Source: three-view drawing plus pictorial views. Frame: mm from the lowest corner of the part. Give positions to 0.01 mm unless a question says otherwise; leave off trailing zeros. Write each loop counter-clockwise with the first axis right and the second up, starting at its lowest first coordinate (ties: lowest second). Pieces come first, ordered by that corner, then holes. Notation, with made-up numbers: M 65,-2.75 L 112,-2.75 A28 ccw 112,23.25 Z; hole C -0.75,69 d11. An arc over 180 degrees is marked long. Return JSON: item names as keys, results as strings.
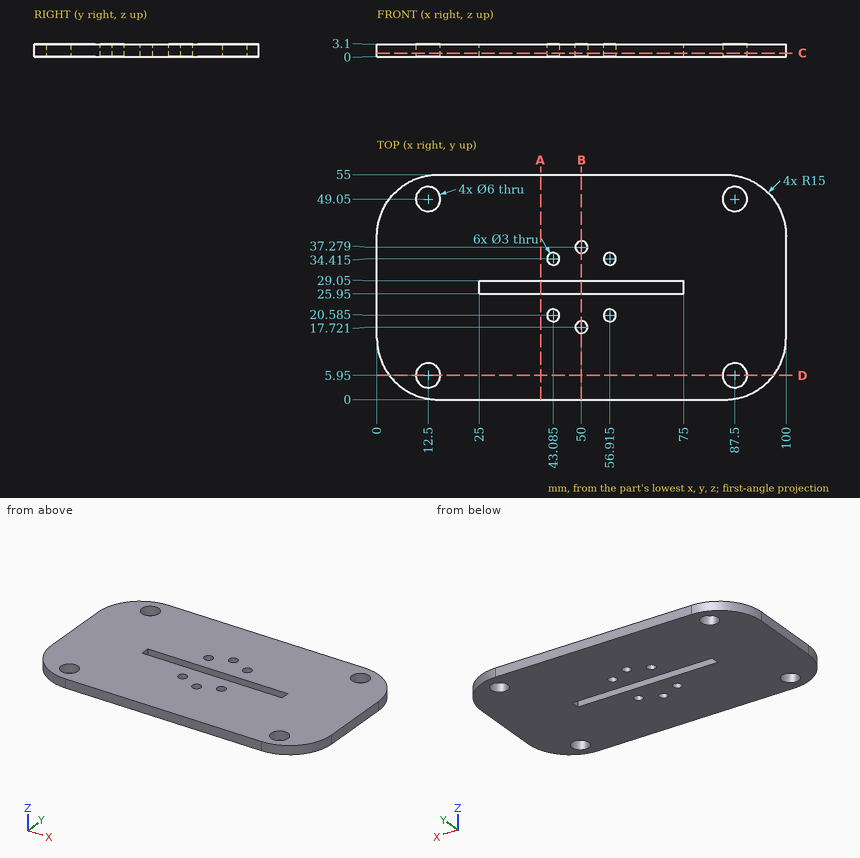
1) Contact query for a flat-ended pin moving along its axis: pin 1 Ø2.5 at (x, y) = (50, 17.721) entering from +Z. Output: stop coordinate, or through.
Numbers:
{"pin 1": "passes through"}
2) Cut plane B-B, the plane x = 50. Return the cut outline in (y, z).
Numbers:
{"outline": "M 0,0 L 16.22,0 L 16.22,3.1 L 0,3.1 Z; M 19.22,0 L 25.95,0 L 25.95,3.1 L 19.22,3.1 Z; M 29.05,0 L 35.78,0 L 35.78,3.1 L 29.05,3.1 Z; M 38.78,0 L 55,0 L 55,3.1 L 38.78,3.1 Z"}
3) Line query: line 1 (Y direction, x = 50, z = 1); line 2 (Y direction, x = 62, z = 0.3); line 3 (Y direction, x = 58, z = 0.55). Output: solid intervals per line, ascending. Write a range as [from, to].
Numbers:
{"line 1": "y = [0, 16.22], [19.22, 25.95], [29.05, 35.78], [38.78, 55]", "line 2": "y = [0, 25.95], [29.05, 55]", "line 3": "y = [0, 19.55], [21.62, 25.95], [29.05, 33.38], [35.45, 55]"}
4) Cut plane C-C, the plane z = 0.85. Give the number of separate pieces and of enclosed holes in the cut face, then the cut area to 3 significant figures.
Numbers:
{"separate pieces": "1", "enclosed holes": "11", "area": "5,000 mm²"}
5) Cut plane A-A, the plane x = 40. Return the cut outline in (y, z).
Numbers:
{"outline": "M 0,0 L 25.95,0 L 25.95,3.1 L 0,3.1 Z; M 29.05,0 L 55,0 L 55,3.1 L 29.05,3.1 Z"}
6) Cut plane D-D, the plane y = 5.95. Return the cut outline in (x, z), then the cut area to 3 significant figures.
Numbers:
{"outline": "M 3.04,0 L 9.5,0 L 9.5,3.1 L 3.04,3.1 Z; M 15.5,0 L 84.5,0 L 84.5,3.1 L 15.5,3.1 Z; M 90.5,0 L 96.96,0 L 96.96,3.1 L 90.5,3.1 Z", "area": "254 mm²"}
